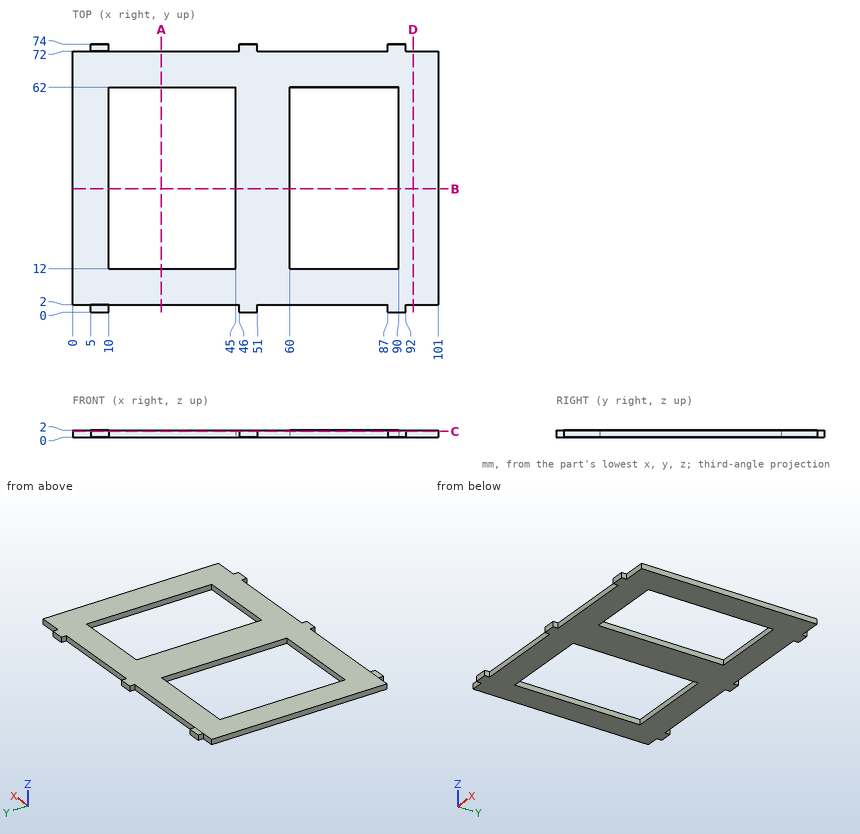
Part print with two shaded views. Sizes in mm from the minimum x, y, z corner. Give positions to 0.01 mm unless a question says otherwise; leave off trailing zeros. Write each loop counter-clockwise with the first axis right and the second up, starting at its lowest first coordinate (ties: lowest second). Pieces come first, ordered by that corner, then holes.
1) Cut at A-A on x = 24.5. Write the cut outline in (y, z).
Resolved:
outline: (2, 0) - (12, 0) - (12, 2) - (2, 2) - close; (62, 0) - (72, 0) - (72, 2) - (62, 2) - close
2) Pin check, flat tips, straight feed: pin 1 (0.6 mm diameter, centred on y = 1.5, z = 1, fed in from -X); pin 2 (0.6 mm diameter, centred on y = 1, z = 1.5, fed in from +X). Stop position of each tip, or through.
Resolved:
pin 1: stops at x = 5
pin 2: stops at x = 92
3) Cut at B-B on y = 34. Write the cut outline in (x, z).
Resolved:
outline: (0, 0) - (10, 0) - (10, 2) - (0, 2) - close; (45, 0) - (60, 0) - (60, 2) - (45, 2) - close; (90, 0) - (101, 0) - (101, 2) - (90, 2) - close
4) Cut at D-D on x = 94. Write the cut outline in (y, z).
Resolved:
outline: (2, 0) - (72, 0) - (72, 2) - (2, 2) - close
5) Probe L1, parallel to X at y = 60.5, z = 1.6; L2, parallel to Y at x = 87.5, z = 1.5; L3, parallel to Y at x = 75, z = 1. List the from-to ranges inside material, lowest first.
Resolved:
L1: x = 0 to 10, 45 to 60, 90 to 101
L2: y = 0 to 12, 62 to 74
L3: y = 2 to 12, 62 to 72
6) Cut at C-C on z = 1.65. State how many separate pieces and enclosed holes the cut face has, then the cut area to 3 significant figures.
Resolved:
separate pieces: 1
enclosed holes: 2
area: 3,880 mm2
